Model file for the job. Use its own axes, mm. A direction names the side the tool comes from. Coordinates: 2 decimals unless noted, no trailing zeros. Write each loop counter-clockwise with the first axis right and the second up, starting at its lowest first coordinate (ties: lowest second). Pieces come first, ordered by that corner, then holes.
Q1. Pull direction Z, two halves, no side cores. Call faces 1 (the flat face through (48, -194, 306)), 2 (the conical face through (18.84, -187.77, 232.68)), 3 (the cylindrical face through (8.58, -191.19, 76.98)), 4 (the cylindrical face through (8.112, -223.106, 196.497)): released by +Z, released by -Z, zero draft, split by the parting line, or undercut.
Q2. Band-saw the part on A-A, the plane x = 31. Write the cut outline in (y, z), plus the area to 3 significant figures.
Q3. Which spindle directions (+Z, -Z, +X, -X, +Y, -Y) get a long thin tool onto all of the face, cutting with end or side? Do faces 5 (the cylindrical face through (35.976, -186.015, 312.424)), 6 (the flat face through (48.9, -210, 85)), 7 (the flat face through (17.4, -188, 67)), 8 (the flat face through (16, -194, 124)). Say none if no direction does.
Q4. Drill centre lines: probe 1 along Y at (x, z) = (9.5, 89); probe 2 along Y at (x, z) = (12.5, 119); probe 3 along Y at (x, z) = (8.5, 28). Where is each one in solid material? Low to high.
Q5. Pin check, flat tips, straight feed: P1, Ø2, axis at y = -384.5, z = 32, coming from the +X side; P2, Ø1, axis at x = 30, y = -409, coming from the +Z side; P3, Ø12, axis at y = -43.5, z = 206.5, coming from the +X side; P4, Ø8, axis at y = -140.5, z = 194, coming from the +X side. Stop position of each tip, or through.
Q6. Band-saw the part on B-B, the plane z = 142.5. State how many separate pieces and enclosed holes the cut face has, plus the area to 3 significant figures.
from build123d import *
from build123d.topology import SkipClean

# Parameters (mm, degrees)
FORO_START              = 60
SKETCH2_R               = 41
FORO_DEPTH              = 120
PATTERNFORI_COUNT       = 8
CUT_EXTRUDE1_DEPTH      = 597.549083718
CUT_EXTRUDE1_DEPTH_BACK = 597.549083718
SKETCH4_W               = 165.941621871
SKETCH4_H               = 884.81830511
CUT_EXTRUDE2_DEPTH      = 597.549083718
CUT_EXTRUDE2_DEPTH_BACK = 597.549083718
SKETCH5_W               = 398.645637441
SKETCH5_H               = 571.659634656


with BuildPart() as part:
    # Sketch1 → Puleggia (revolve)
    with BuildSketch(Plane.XY, mode=Mode.PRIVATE) as puleggia_sk:
        with BuildLine():
            Line((14.305754261, 90.102284872), (23.610406599, 119.612871865))
            Line((23.610406599, 119.612871865), (48, 119.612871865))
            Line((48, 119.612871865), (48, 108.49032691))
            ThreePointArc((48, 108.49032691), (41.937089486, 106.505733817), (38.221197059, 101.320211941))
            Line((38.221197059, 101.320211941), (17.85132197, 36.715221983))
            ThreePointArc((17.85132197, 36.715221983), (16.465539581, 30.77192545), (16, 24.686990003))
            Line((16, 24.686990003), (16, -72.887128135))
            ThreePointArc((16, -72.887128135), (18.343145751, -78.543982385), (24, -80.887128135))
            Line((24, -80.887128135), (48.9, -80.887128135))
            Line((48.9, -80.887128135), (48.9, -115.887128135))
            Line((48.9, -115.887128135), (0, -115.887128135))
            Line((0, -115.887128135), (0, 79.612871865))
            ThreePointArc((0, 79.612871865), (8.869644725, 82.516202801), (14.305754261, 90.102284872))
        make_face()
    puleggia = revolve(puleggia_sk.sketch.rotate(Axis((-62.254886415, -192.887128135, 0), (1, 0, 0)), 90), axis=Axis((-62.254886415, -192.887128135, 0), (1, 0, 0)))

    # Mirror 2: Puleggia across plane
    with SkipClean():  # the faces are left unmerged after this step: merging them gives an invalid solid
        add(puleggia.mirror(Plane(origin=(0, 79.612871865, 0), x_dir=(0, 0, 1), z_dir=(1, 0, 0))))

    # Sketch2 → Foro (cut)
    with SkipClean():  # the faces are left unmerged after this step: merging them gives an invalid solid
        with BuildSketch(Plane(origin=(0, 0, 0), x_dir=(0, 0, -1), z_dir=(1, 0, 0)).offset(FORO_START)):
            with Locations((0, -24.100069066)):
                Circle(SKETCH2_R)
        foro = extrude(amount=-FORO_DEPTH, mode=Mode.SUBTRACT)

    # PatternFori: Foro ×8 about axis
    with SkipClean():  # the faces are left unmerged after this step: merging them gives an invalid solid
        patternfori_axis = Axis((0, -192.887128135, 0), (1, 0, 0))
        for i in range(1, PATTERNFORI_COUNT):
            add(foro.rotate(patternfori_axis, i * 360 / PATTERNFORI_COUNT), mode=Mode.SUBTRACT)

    # Sketch3 → Revolve1 (revolve)
    with SkipClean():  # the faces are left unmerged after this step: merging them gives an invalid solid
        with BuildSketch(Plane.XY, mode=Mode.PRIVATE) as revolve1_sk:
            Polygon((48.9, -115.887128135), (48.9, -107.887128135), (52.9, -107.887128135), (52.9, -127.887128135), (48.203298426, -127.887128135), (17.4, -127.887128135), (17.4, -115.887128135), align=None)
        revolve1 = revolve(revolve1_sk.sketch.rotate(Axis((48.9, -192.887128135, 0), (-1, 0, 0)), 90), axis=Axis((48.9, -192.887128135, 0), (-1, 0, 0)))

    # Mirror1: Revolve1 across plane
    with SkipClean():  # the faces are left unmerged after this step: merging them gives an invalid solid
        add(revolve1.mirror(Plane(origin=(0, 0, 0), x_dir=(0, 0, 1), z_dir=(1, 0, 0))))

    # Sketch4 → Cut-Extrude1 (cut, two sides: drawn at the far end of the back side and taken through both)
    with BuildSketch(Plane.XY.offset(-CUT_EXTRUDE1_DEPTH_BACK)):
        with Locations((-82.970810936, -207.065039304)):
            Rectangle(SKETCH4_W, SKETCH4_H)
    extrude(amount=CUT_EXTRUDE1_DEPTH + CUT_EXTRUDE1_DEPTH_BACK, mode=Mode.SUBTRACT)

    # Sketch5 → Cut-Extrude2 (cut, two sides: drawn at the far end of the back side and taken through both)
    with BuildSketch(Plane(origin=(0, 0, 0), x_dir=(1, 0, 0), z_dir=(0, 1, 0)).offset(-CUT_EXTRUDE2_DEPTH_BACK)):
        with Locations((15.58753589, 285.829817328)):
            Rectangle(SKETCH5_W, SKETCH5_H)
    extrude(amount=CUT_EXTRUDE2_DEPTH + CUT_EXTRUDE2_DEPTH_BACK, mode=Mode.SUBTRACT)


solid = part.part
Answer sheet:
1. face 1: zero draft
1. face 2: undercut
1. face 3: released by -Z
1. face 4: undercut
2. outline: (-505.39, 0) - (-464.19, 0) arc R271.3 cw to (78.42, 0) - (119.61, 0) arc R312.5 ccw to start; (-304.89, 0) - (-257.89, 0) arc R65 cw to (-127.89, 0) - (-80.89, 0) arc R112 ccw to start
2. area: 50,800 mm2
3. face 5: +Z, +X, -X
3. face 6: +Z, +X
3. face 7: -Z, -X
3. face 8: +X
4. probe 1: y = -454.03 to -339.8, -284.67 to -101.1, -45.97 to 68.26
4. probe 2: y = -445.47 to -353.24, -271.24 to -114.54, -32.54 to 59.69
4. probe 3: y = -466.6 to -391.62, -331.72 to -264.62, -121.16 to -54.05, 5.85 to 80.83
5. P1: passes through
5. P2: stops at z = 226.2
5. P3: stops at x = 27.71
5. P4: stops at x = 16
6. separate pieces: 4
6. enclosed holes: 0
6. area: 7,260 mm2
